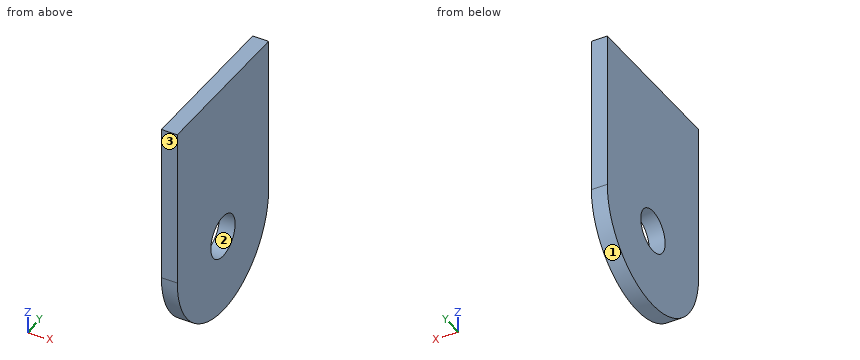
Autodesk Inventor part; units mm, degrees
ref_plane "YZ Plane" through (0, 0, 0) normal (1, 0, 0) x (0, 1, 0)
ref_plane "XZ Plane" through (0, 0, 0) normal (0, 1, 0) x (-1, 0, 0)
ref_plane "XY Plane" through (0, 0, 0) normal (0, 0, 1) x (1, 0, 0)
sketch "Boceto1" plane through (0, 0, 0) normal (1, 0, 0) x (0, 1, 0)
  line L0 (0, 0) -> (-30, 0)
  line L1 (-30, 0) -> (-30, -30)
  line L2 (-30, -30) -> (0, -30)
  line L3 (0, -30) -> (0, 0)
  circle A0 centre (-15, -30) radius 15
  dimension "d0" = 30
  dimension "d1" = 30
  dimension "d2" = 30
  dimension "d3" = 15
extrude "Extrusión1" add sketch "Boceto1" along normal blind 3
sketch "Boceto2" plane through (0, 0, 0) normal (-1, 0, 0) x (0, 0, 1)
  arc A0 (-30, 0) -> (-30, -30) centre (-30, -15) ccw
  circle A1 centre (-30, -15) radius 4
  point P0 (0, 0)
  dimension "d6" = 8
extrude "Extrusión2" cut sketch "Boceto2" against normal blind 5
properties part number "soporte vertical"
The listing builds one solid part. Answer for the finished solid, in the listing's coordinates (mm). Face numbers are marked on the shaded views. Coordinates: 2 decimals unless noted, no trailing zeros. Loops run counter-clockwise (first coordinate to the right, second up) from the corner with the lowest first, then second, coordinate; pieces in that order, holes last. Notation, with made-up numbers: (45, 74.25) -> (99, 74.25) arc R26 cw to (99, 89.25) -> close; hole circle Ø1 at (83.5, -2). An arc over 180 degrees is marked (long way). Write item = value, one per line. Start each with the question number.
1) A cutting plane is placed at D-D (y = -22.5). Give the vertices of the cut face in (x, z).
2) A cutting plane is placed at A-A (y = -15). Give the vertices of the cut face in (x, z), then the cut area to 3 significant figures.
3) A cutting plane is placed at B-B (z = -29.5). Give the vertices of the cut face in (x, y), then the cut area to 3 significant figures.
4) A cutting plane is placed at C-C (x = 2). Give the vertices of the cut face in (y, z).
5) Straight lines are drawn through the part: line 1 (Y direction, x = 1.95, z = -30); line 2 (Z direction, x = 0.75, y = -17.5); line 3 (Z direction, x = 2.9, y = -12). For each, find the intervals that lie inside material, in ascending order. Write a range as from..to.
6) The mould has two halves that part along Z. Classify the marked faces 1, 2 and 3: released by +Z, released by -Z, zero draft, split by the parting line, or undercut.
Responses:
q1.outline = (0, -42.99) -> (3, -42.99) -> (3, 0) -> (0, 0) -> close
q2.outline = (0, -45) -> (3, -45) -> (3, -34) -> (0, -34) -> close; (0, -26) -> (3, -26) -> (3, 0) -> (0, 0) -> close
q2.area = 111 mm²
q3.outline = (0, -30) -> (3, -30) -> (3, -18.97) -> (0, -18.97) -> close; (0, -11.03) -> (3, -11.03) -> (3, 0) -> (0, 0) -> close
q3.area = 66.2 mm²
q4.outline = (-30, -30) arc R15 ccw to (0, -30) -> (0, 0) -> (-30, 0) -> close; hole circle Ø8 at (-15, -30)
q5.line_1 = -30..-19, -11..0
q5.line_2 = -44.79..-33.12, -26.88..0
q5.line_3 = -44.7..-32.65, -27.35..0
q6.face_1 = released by -Z
q6.face_2 = undercut
q6.face_3 = zero draft
